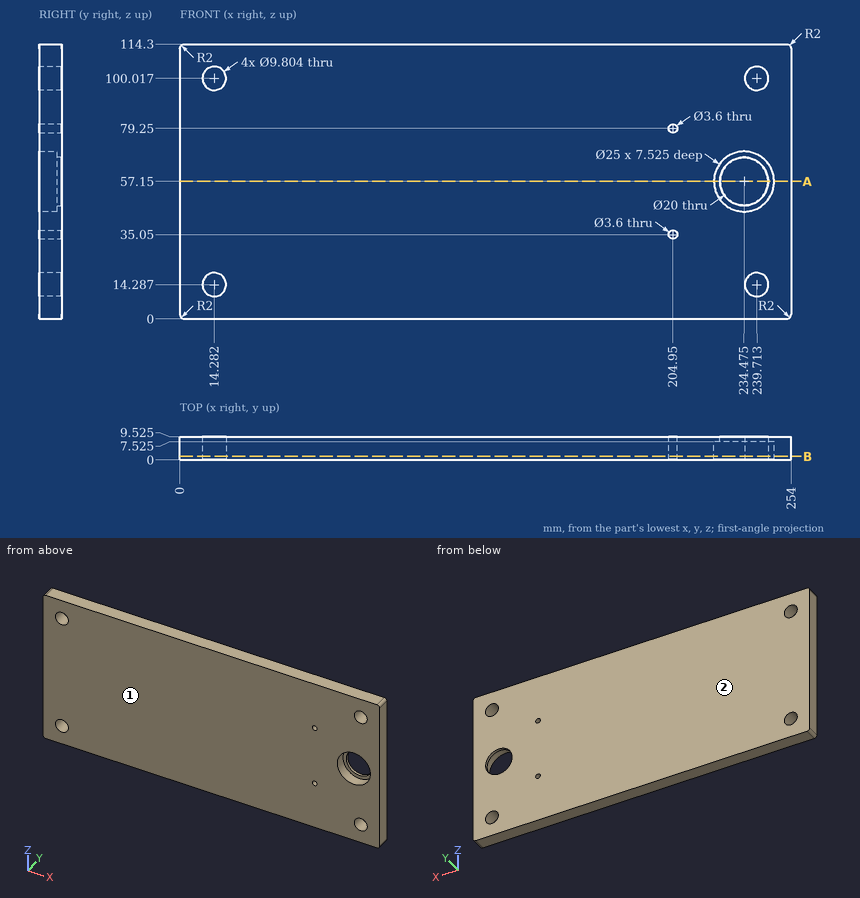
The drawing under review shows one solid part. Ordinate dimensions are in mm from its lowest x, y, z. Round coordinates to 2 decimals unless told otherwise and drop trailing zeros. Loops run counter-clockwise (first coordinate to the right, second up) from the corner with the lowest first, then second, coordinate; pieces in that order, holes last. Notation, with made-up numbers: (42, 86.5) - (47, 86.5) arc R30 cw to (47, 122.5) - close; hole circle Ø4 at (-34.5, -35.5). An arc over 180 degrees is marked (long way). Use a Markdown table: item, result. Add a question column.
Q1. Add section A-A (z = 57.15). State the section outline as (x, y) points (1 decimal).
Q2. The part is to be moulded in two halves that separate along Y. For the marked faces 1 and 2, say which applies: pulls with the +Y half, pulls with the -Y half, needs draft (parallel to the pull), parting line crosses it, or undercut.
Q3. Insertion check: pin 1 Ø15.5 at (x, z) = (14.28, 100.02) entering from -Y. The pin has a flat end and moves straight along its axis. Give the tip position at first contact, or say it passes through.
Q4. Add section B-B (y = 1.5). State how many separate pieces and enclosed holes the cut face has, plus the area to 3 significant figures.
Q5. For probe 1 along X at (y, z) = (8.5, 100.5) (1 decimal); probe 2 along Z at (x, y) = (204.95, 5); probe 3 along X at (y, z) = (9.25, 55), list the stretches that pass through material, from the lowest coordinate up.
Worked answers:
| question | item | result |
|---|---|---|
| 1 | outline | (0, 0) - (222, 0) - (222, 7.5) - (224.5, 7.5) - (224.5, 9.5) - (0, 9.5) - close; (244.5, 7.5) - (247, 7.5) - (247, 0) - (254, 0) - (254, 9.5) - (244.5, 9.5) - close |
| 2 | face 1 | pulls with the -Y half |
| 2 | face 2 | pulls with the +Y half |
| 3 | pin 1 | y = 0 |
| 4 | separate pieces | 1 |
| 4 | enclosed holes | 7 |
| 4 | area | 28,200 mm² |
| 5 | probe 1 | 0 to 9.4, 19.2 to 234.8, 244.6 to 254 |
| 5 | probe 2 | 0 to 33.25, 36.85 to 77.45, 81.05 to 114.3 |
| 5 | probe 3 | 0 to 224.71, 244.24 to 254 |
